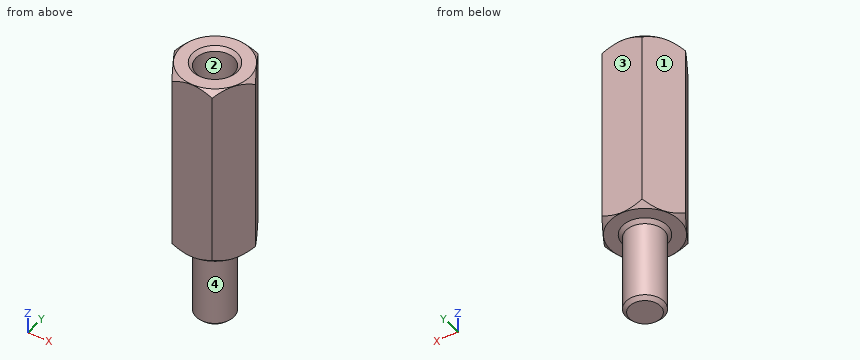
from build123d import *

# Parameters (mm, degrees)
HEX_2_DEPTH                 = 6.675
TAP_DRILL_FOR_M3X0_5_TAP1_D = 2.7
THREAD_DEPTH                = 6
THREAD_DEPTH_BACK           = 2
SKETCH8_R                   = 1.35
INNERCHAMFER_SIZE           = 0.25


with BuildPart() as part:
    # Sketch1 → HEX 2 (new, symmetric)
    with BuildSketch(Plane.XY):
        Polygon((2.886751346, 0), (1.443375673, 2.5), (-1.443375673, 2.5), (-2.886751346, 0), (-1.443375673, -2.5), (1.443375673, -2.5), align=None)
    extrude(amount=HEX_2_DEPTH, both=True)

    # Tap Drill for M3x0.5 Tap1 (through all)
    with Locations(Plane.XY.offset(6.675)):
        with Locations((0, 0)):
            Hole(TAP_DRILL_FOR_M3X0_5_TAP1_D / 2)

    # Sketch7 → HexChamfer (revolve, cut)
    with BuildSketch(Plane(origin=(0, 0, 0), x_dir=(1, 0, 0), z_dir=(0, 1, 0)), mode=Mode.PRIVATE) as hexchamfer_sk:
        Polygon((-2.886751346, 6.675), (-2.886751346, 6.275), (-2.486751346, 6.675), align=None)
    hexchamfer = revolve(hexchamfer_sk.sketch.rotate(Axis((0, 0, 15.266742202), (0, 0, -1)), 180), axis=Axis((0, 0, 15.266742202), (0, 0, -1)), mode=Mode.SUBTRACT)

    # Mirror1: HexChamfer across plane
    add(hexchamfer.mirror(Plane.XY), mode=Mode.SUBTRACT)

    # Sketch8 → Thread (add, two sides: drawn at the far end of the back side and taken through both)
    with BuildSketch(Plane(origin=(0, 0, -6.675), x_dir=(-1, 0, 0), z_dir=(0, 0, -1)).offset(-THREAD_DEPTH_BACK)):
        with Locations(Location((0, 0, 0), (0, 0, 180))):
            Circle(SKETCH8_R)
    extrude(amount=THREAD_DEPTH + THREAD_DEPTH_BACK)

    # InnerChamfer
    innerchamfer_edges = [part.edges().sort_by_distance(p)[0] for p in [
        (1.35, 0, 6.675),
        (-1.35, 0, -6.675),
        (-1.35, 0, -12.675),
    ]]
    chamfer(innerchamfer_edges, length=INNERCHAMFER_SIZE)


solid = part.part
CAD build for the part. Positions are in the model's coordinates, mm. Face numbers are marked on the shaded views. Coordinates: 2 decimals unless noted, no trailing zeros. Write each loop counter-clockwise with the first axis right and the second up, starting at its lowest first coordinate (ties: lowest second). Pieces come first, ordered by that corner, then holes. Notation, with made-up numbers: (-20, 1) - (29, 1) arc R11 ccw to (29, 15) - close; hole circle Ø9 at (62.25, -2). An arc over 180 degrees is marked (long way). Use a Markdown table: item, result. Add a question column.
Item 1: Drill centre lines: L1, parallel to Y at x = 0, z = 4; L2, parallel to Z at x = 1.2, y = -1.45 (3 decimals); L3, parallel to X at y = 0.35, z = 3.75. Where is each one in solid material? Low to high. Write a range as from..to.
Item 2: Band-saw the part on C-C, the plane z = -10.5. Give the cut face in (x, y).
Item 3: Band-saw the part on A-A, the plane z = 4. Give the cut face in (x, y), and give its area (3 significant figures).
Item 4: Band-saw the part on B-B, the plane x = 0. Give the cut face in (y, z) (3 decimals), and give its area (3 significant figures).
Item 5: Mould opens along X. For the marked faces 1, 2, 3 and 4 say: pulls with the +X half, pulls with the -X half, needs draft (parallel to the pull), parting line crosses it, or undercut.
Numbers:
| question | item | result |
|---|---|---|
| 1 | L1 | -2.5..-1.35, 1.35..2.5 |
| 1 | L2 | -6.675..6.675 |
| 1 | L3 | -2.68..-1.3, 1.3..2.68 |
| 2 | outline | circle Ø2.7 at (0, 0) |
| 3 | outline | (-2.89, 0) - (-1.44, -2.5) - (1.44, -2.5) - (2.89, 0) - (1.44, 2.5) - (-1.44, 2.5) - close; hole circle Ø2.7 at (0, 0) |
| 3 | area | 15.9 mm2 |
| 4 | outline | (-2.5, -6.662) - (-2.487, -6.675) - (-1.6, -6.675) - (-1.35, -6.925) - (-1.35, -12.425) - (-1.1, -12.675) - (1.1, -12.675) - (1.35, -12.425) - (1.35, -6.925) - (1.6, -6.675) - (2.487, -6.675) - (2.5, -6.662) - (2.5, 6.662) - (2.487, 6.675) - (1.6, 6.675) - (1.35, 6.425) - (1.35, -4.675) - (-1.35, -4.675) - (-1.35, 6.425) - (-1.6, 6.675) - (-2.487, 6.675) - (-2.5, 6.662) - close |
| 4 | area | 52.2 mm2 |
| 5 | face 1 | pulls with the -X half |
| 5 | face 2 | undercut |
| 5 | face 3 | needs draft |
| 5 | face 4 | parting line crosses it |
